The listing builds one solid part. Answer for the finished solid, in the listing's coordinates (mm). A direction names the side the tool comes from. Round coordinates to 2 decimals unless told otherwise and drop trailing zeros. Loops run counter-clockwise (first coordinate to the right, second up) from the corner with the lowest first, then second, coordinate; pieces in that order, holes last. Notation, with made-up numbers: (-33, -36) - (-1, -36) arc R31 cw to (-1, -5) - close; hole circle Ø4 at (74.25, -19). An arc over 180 degrees is marked (long way). One line per question, with ' | ' between items. Start each with the question number.
from build123d import *

# Parameters (mm, degrees)
BASE_FLANGE1_DEPTH       = 50
M4_START                 = -1.5
M4_CLEARANCE_SLOT1_DEPTH = 1.5
M4_CLEARANCE_HOLE1_D     = 4.5
FILLET1_R                = 5


# Read off the part's stored shape, not the designer's step: M4 Clearance Slot1
# Sheet-metal steps are written as plain solids
with BuildPart() as part:
    # Sketch1 → Base-Flange1 (new body)
    with BuildSketch(Plane.XY):
        with BuildLine():
            Line((73, 0), (3, 0))
            ThreePointArc((3, 0), (0.878679656, -0.878679656), (0, -3))
            Line((0, -3), (0, -30))
            Line((0, -30), (1.5, -30))
            Line((1.5, -30), (1.5, -3))
            ThreePointArc((1.5, -3), (1.939339828, -1.939339828), (3, -1.5))
            Line((3, -1.5), (73, -1.5))
            Line((73, -1.5), (73, 0))
        make_face()
    extrude(amount=BASE_FLANGE1_DEPTH)

    # M4 Clearance Slot1 outline → M4 Clearance Slot1 (cut)
    with BuildSketch(Plane(origin=(0, 0, 0), x_dir=(1, 0, 0), z_dir=(0, 1, 0)).offset(M4_START)):
        with BuildLine():
            Line((47.15, -40.25), (47.15, -29.75))
            ThreePointArc((47.15, -29.75), (44.9, -27.5), (42.65, -29.75))
            Line((42.65, -29.75), (42.65, -40.25))
            ThreePointArc((42.65, -40.25), (44.9, -42.5), (47.15, -40.25))
        make_face()
        with BuildLine():
            Line((67.15, -40.25), (67.15, -29.75))
            ThreePointArc((67.15, -29.75), (64.9, -27.5), (62.65, -29.75))
            Line((62.65, -29.75), (62.65, -40.25))
            ThreePointArc((62.65, -40.25), (64.9, -42.5), (67.15, -40.25))
        make_face()
    extrude(amount=M4_CLEARANCE_SLOT1_DEPTH, mode=Mode.SUBTRACT)

    # M4 Clearance Hole1 (through all)
    with Locations(Plane(origin=(1.5, 0, 0), x_dir=(0, 0, -1), z_dir=(1, 0, 0))):
        with Locations((-40, -16.5), (-10, -16.5)):
            Hole(M4_CLEARANCE_HOLE1_D / 2)

    # Fillet1
    fillet1_edges = [part.edges().sort_by_distance(p)[0] for p in [
        (73, -0.75, 50),
        (73, -0.75, 0),
        (0.75, -30, 50),
        (0.75, -30, 0),
    ]]
    fillet(fillet1_edges, radius=FILLET1_R)


solid = part.part
(1) A tool of negligible diameter and unlimited length cuts with its end or side. For faces 5 (the cylindrical face through (44.9, -0.8, 27.5)), 6 (the cylindrical face through (72, -1, 2)), 7 (the flat face through (1.5, -17, 25)), from which of +Z, -Z, +X, -X, +Y, -Y can it reach the whole face along a straight path? Write none if from no direction.
(2) Determine the mould class of faces 1 (the cylindrical face through (72, -1, 48)), 2 (the flat face through (24, -1, 0)), 3 (the flat face through (47.15, -1, 35)), 4 (the flat face through (0, -16, 25)) for opening direction Z: pulls with the +Z half, pulls with the -Z half, needs draft (parallel to the pull), parting line crosses it, or undercut.
(3) Find section C-C on z = 10. Write down the section's boundary in (x, y).
(4) Find section A-A on x = 64.9. Write down the section's boundary in (y, z), plus the area to 3 significant figures.
(5) Find section D-D on z = 24. Write down the section's boundary in (x, y).
(6) Consider L1, parallel to Y at x = 59, z = 11; L2, parallel to X at y = -20.5, z = 42.5; L3, parallel to Y at x = 0.85, z = 40. Determine where each line is inside the solid, lowest interval first.
(7) Find section B-B on z = 36. Write down the section's boundary in (x, y), plus the area to 3 significant figures.
(8) Each of these flat-tipped pins is pushed along its axis until it touches: P1, Ø5, axis at y = -17.5, z = 38, coming from the +X side; P2, Ø3, axis at x = 50.5, z = 31, coming from the -Y side; P3, Ø1.6, axis at y = -1, z = 33, coming from the -X side. Where does it stop, or does it pass through?
Answer below:
1) face 5: +Y, -Y | face 6: -Z, +X, +Y, -Y | face 7: +Z, -Z, +X, -Y
2) face 1: pulls with the +Z half | face 2: pulls with the -Z half | face 3: undercut | face 4: needs draft
3) outline: (0, -30) - (1.5, -30) - (1.5, -18.75) - (0, -18.75) - close; (0, -14.25) - (1.5, -14.25) - (1.5, -3) arc R1.5 cw to (3, -1.5) - (73, -1.5) - (73, 0) - (3, 0) arc R3 ccw to (0, -3) - close
4) outline: (-1.5, 0) - (0, 0) - (0, 27.5) - (-1.5, 27.5) - close; (-1.5, 42.5) - (0, 42.5) - (0, 50) - (-1.5, 50) - close | area: 52.5 mm2
5) outline: (0, -30) - (1.5, -30) - (1.5, -3) arc R1.5 cw to (3, -1.5) - (73, -1.5) - (73, 0) - (3, 0) arc R3 ccw to (0, -3) - close
6) L1: -1.5 to 0 | L2: 0 to 1.5 | L3: -30 to -18.75, -14.25 to -0.91
7) outline: (0, -30) - (1.5, -30) - (1.5, -3) arc R1.5 cw to (3, -1.5) - (42.65, -1.5) - (42.65, 0) - (3, 0) arc R3 ccw to (0, -3) - close; (47.15, -1.5) - (62.65, -1.5) - (62.65, 0) - (47.15, 0) - close; (67.15, -1.5) - (73, -1.5) - (73, 0) - (67.15, 0) - close | area: 137 mm2
8) P1: x = 1.5 | P2: y = -1.5 | P3: x = 0.25
